The model under review builds one solid part; all positions refer to its coordinate system, in mm. Face numbers are marked on the shaded views. A direction names the side the tool comes from. Round coordinates to 2 decimals unless told otherwise and drop trailing zeros. Loops run counter-clockwise (first coordinate to the right, second up) from the corner with the lowest first, then second, coordinate; pieces in that order, holes last. Notation, with made-up numbers: (-26.5, 49) - (-11.5, 49) arc R30 ccw to (-11.5, 72) - close; hole circle Ø7 at (51, 46). An arc over 180 degrees is marked (long way). Answer as CSV lines item,"result".
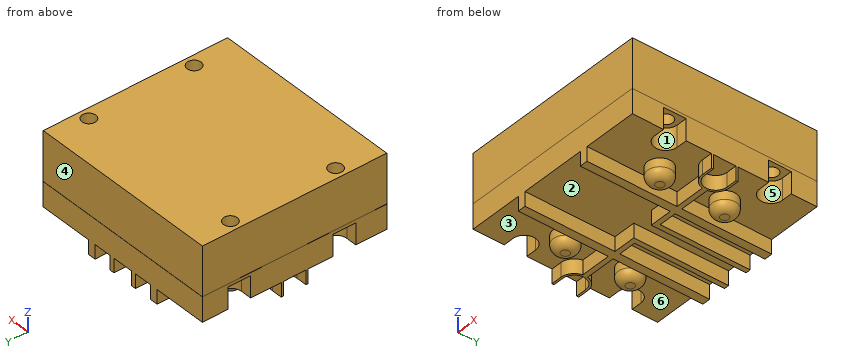
from build123d import *

# Parameters (mm, degrees)
SKETCH1_W           = 59.9948
SKETCH1_H           = 57.9628
BOSS_EXTRUDE1_DEPTH = 27.4828
SKETCH2_R           = 2.1463
CUT_EXTRUDE1_DEPTH  = 50.950674155
CUT_EXTRUDE2_DEPTH  = 11.176
SKETCH4_W           = 5.588
SKETCH4_H           = 28.2194
CUT_EXTRUDE3_DEPTH  = 4.445
SKETCH5_W           = 59.9948
SKETCH5_H           = 57.9628
SKETCH5_W_2         = 59.944
SKETCH5_H_2         = 57.8612
CUT_EXTRUDE4_DEPTH  = 15.367
SKETCH6_R           = 3.81
BOSS_EXTRUDE2_DEPTH = 5.207
FILLET1_R           = 2.54


with BuildPart() as part:
    # Sketch1 → Boss-Extrude1 (new body)
    with BuildSketch(Plane.XY):
        Rectangle(SKETCH1_W, SKETCH1_H)
    extrude(amount=BOSS_EXTRUDE1_DEPTH)

    # Sketch2 → Cut-Extrude1 (cut, through all)
    with BuildSketch(Plane.XY.offset(27.4828)):
        with Locations((-26.6446, -15.6464)):
            Circle(SKETCH2_R)
        with Locations((-26.6446, 17.3736)):
            Circle(SKETCH2_R)
    cut_extrude1 = extrude(amount=-CUT_EXTRUDE1_DEPTH, mode=Mode.SUBTRACT)

    # Mirror1: Cut-Extrude1 across plane
    add(cut_extrude1.mirror(Plane(origin=(0, 0, 0), x_dir=(0, 0, 1), z_dir=(1, 0, 0))), mode=Mode.SUBTRACT)

    # Sketch3 → Cut-Extrude2 (cut)
    with BuildSketch(Plane(origin=(0, 0, 0), x_dir=(-1, 0, 0), z_dir=(0, 0, -1))):
        with BuildLine():
            Line((-26.6446, 20.9296), (-29.9974, 20.9296))
            Line((-29.9974, 20.9296), (-29.9974, 13.8176))
            Line((-29.9974, 13.8176), (-26.6446, 13.8176))
            ThreePointArc((-26.6446, 13.8176), (-23.0886, 17.3736), (-26.6446, 20.9296))
        make_face()
        with BuildLine():
            Line((-26.6446, -12.0904), (-29.9974, -12.0904))
            Line((-29.9974, -12.0904), (-29.9974, -19.2024))
            Line((-29.9974, -19.2024), (-26.6446, -19.2024))
            ThreePointArc((-26.6446, -19.2024), (-23.0886, -15.6464), (-26.6446, -12.0904))
        make_face()
        with BuildLine():
            Line((26.6446, 20.9296), (29.9974, 20.9296))
            Line((29.9974, 20.9296), (29.9974, 13.8176))
            Line((29.9974, 13.8176), (26.6446, 13.8176))
            ThreePointArc((26.6446, 13.8176), (23.0886, 17.3736), (26.6446, 20.9296))
        make_face()
        with BuildLine():
            Line((26.6446, -12.0904), (29.9974, -12.0904))
            Line((29.9974, -12.0904), (29.9974, -19.2024))
            Line((29.9974, -19.2024), (26.6446, -19.2024))
            ThreePointArc((26.6446, -19.2024), (23.0886, -15.6464), (26.6446, -12.0904))
        make_face()
    extrude(amount=-CUT_EXTRUDE2_DEPTH, mode=Mode.SUBTRACT)

    # Sketch4 → Cut-Extrude3 (cut)
    with BuildSketch(Plane(origin=(0, 0, 0), x_dir=(-1, 0, 0), z_dir=(0, 0, -1))):
        with BuildLine():
            ThreePointArc((22.518386513, 0.762), (23.960485441, 3.225183836), (26.6446, 4.195984001))
            Line((26.6446, 4.195984001), (29.9974, 4.195984001))
            Line((29.9974, 4.195984001), (29.9974, 28.9814))
            Line((29.9974, 28.9814), (12.954, 28.9814))
            Line((12.954, 28.9814), (12.954, 0.762))
            Line((12.954, 0.762), (22.518386513, 0.762))
        make_face()
        with BuildLine():
            Line((29.9974, -28.9814), (29.9974, -4.195984001))
            Line((29.9974, -4.195984001), (26.6446, -4.195984001))
            ThreePointArc((26.6446, -4.195984001), (23.960485441, -3.225183836), (22.518386513, -0.762))
            Line((22.518386513, -0.762), (12.954, -0.762))
            Line((12.954, -0.762), (12.954, -28.9814))
            Line((12.954, -28.9814), (29.9974, -28.9814))
        make_face()
        with BuildLine():
            Line((29.9974, -3.556), (29.9974, 3.556))
            Line((29.9974, 3.556), (26.6446, 3.556))
            ThreePointArc((26.6446, 3.556), (23.0886, 0), (26.6446, -3.556))
            Line((26.6446, -3.556), (29.9974, -3.556))
        make_face()
        Polygon((0, -28.9814), (10.414, -28.9814), (10.414, -0.762), (3.302, -0.762), (3.302, 28.9814), (0, 28.9814), align=None)
        with Locations((7.62, 14.8717)):
            Rectangle(SKETCH4_W, SKETCH4_H)
    cut_extrude3 = extrude(amount=-CUT_EXTRUDE3_DEPTH, mode=Mode.SUBTRACT)

    # Mirror2: Cut-Extrude3 across plane
    add(cut_extrude3.mirror(Plane(origin=(0, 0, 0), x_dir=(0, 0, 1), z_dir=(1, 0, 0))), mode=Mode.SUBTRACT)

    # Sketch5 → Cut-Extrude4 (cut)
    with BuildSketch(Plane.XY.offset(27.4828)):
        Rectangle(SKETCH5_W, SKETCH5_H)
        Rectangle(SKETCH5_W_2, SKETCH5_H_2, mode=Mode.SUBTRACT)
    extrude(amount=-CUT_EXTRUDE4_DEPTH, mode=Mode.SUBTRACT)

    # Sketch6 → Boss-Extrude2 (add)
    with BuildSketch(Plane(origin=(0, 0, 4.445), x_dir=(-1, 0, 0), z_dir=(0, 0, -1))):
        with Locations((-17.78, 10.16)):
            Circle(SKETCH6_R)
        with Locations((17.78, 10.16)):
            Circle(SKETCH6_R)
        with Locations((17.78, -10.16)):
            Circle(SKETCH6_R)
        with Locations((-17.78, -10.16)):
            Circle(SKETCH6_R)
    extrude(amount=BOSS_EXTRUDE2_DEPTH)

    # Fillet1
    fillet1_edges = [part.edges().sort_by_distance(p)[0] for p in [
        (21.59, 10.16, -0.762),
        (-13.97, 10.16, -0.762),
        (-13.97, -10.16, -0.762),
        (21.59, -10.16, -0.762),
    ]]
    fillet(fillet1_edges, radius=FILLET1_R)


solid = part.part
1. Take a section at B-B (y = 0). State the section outline as (x, z) points (3 decimals), plus the area to 3 significant figures.
Numbers:
outline,"(-29.997, 4.445) - (-23.089, 4.445) - (-23.089, 0) - (-3.302, 0) - (-3.302, 4.445) - (3.302, 4.445) - (3.302, 0) - (23.089, 0) - (23.089, 4.445) - (29.997, 4.445) - (29.997, 12.116) - (29.972, 12.116) - (29.972, 27.483) - (-29.972, 27.483) - (-29.972, 12.116) - (-29.997, 12.116) - close"
area,"1,560 mm²"
2. Wall thickness on probe 1 along X at (y, z) = (-14, 18.25); probe 2 along Y at (x, z) = (-21, 1.25); probe 3 along Y at (x, z) = (20, 2): over which ranges is each line inside the solid? List them lowest first.
Numbers:
probe 1,"x = -29.97 to -28.02, -25.27 to 25.27, 28.02 to 29.97"
probe 2,"y = -12.09 to -8.23, -0.76 to 0.76, 8.23 to 12.09"
probe 3,"y = -13.26 to -7.06, -0.76 to 0.76, 7.06 to 13.26"
3. Draft analysis for pull direction Y (two halves, no side actions). For the marked faces 1, 2, 3 and 4, state which applies: +Y half, -Y half, draft (parallel to the pull), parting line (faces both ways), or undercut.
Numbers:
face 1,"undercut"
face 2,"draft"
face 3,"undercut"
face 4,"+Y half"
4. Take a section at A-A (x = -6). State the section outline as (y, z) points (3 decimals).
Numbers:
outline,"(-28.981, 4.445) - (-0.762, 4.445) - (-0.762, 0) - (0.762, 0) - (0.762, 4.445) - (28.981, 4.445) - (28.981, 12.116) - (28.931, 12.116) - (28.931, 27.483) - (-28.931, 27.483) - (-28.931, 12.116) - (-28.981, 12.116) - close"
5. Clearance check with flat-ended pins moving along their axes: pin 1 (5 mm diameter, centred on x = 21.5, y = 2.5, fed in from -Z); pin 2 (1 mm diameter, centred on x = -28.5, z = 3, fed in from +Y); pin 3 (8 mm diameter, centred on x = -0.5, y = -13, fed in from -Z) (3 decimals). State where each tip first meets the part, or that it passes through.
Numbers:
pin 1,"stops at z = 0"
pin 2,"stops at y = 4.2"
pin 3,"stops at z = 4.445"
6. Take a section at D-D (z = 16.25). State the section outline as (x, y) points.
Numbers:
outline,"(-29.97, -28.93) - (29.97, -28.93) - (29.97, 28.93) - (-29.97, 28.93) - close; hole circle Ø4.29 at (-26.64, -15.65); hole circle Ø4.29 at (-26.64, 17.37); hole circle Ø4.29 at (26.64, -15.65); hole circle Ø4.29 at (26.64, 17.37)"
7. Take a section at C-C (x = 25.5). State how many separate pieces and enclosed holes the cut face has, plus the area to 3 significant figures.
Numbers:
separate pieces,"3"
enclosed holes,"0"
area,"1,130 mm²"
8. Tool access review of the marked faces 5 and 6: name each direction out of +Z, -Z, +X, -X, +Y, -Y from which nothing blocks a thin tool from reaching the whole face with its end or side.
Numbers:
face 5,"-Z, +X"
face 6,"-Z"
